Geometry check sheet. Reference: the model listing, model coordinates, mm. A direction names the side the tool comes from. Round coordinates to 2 decimals unless told otherwise and drop trailing zeros. Write each loop counter-clockwise with the first axis right and the second up, starting at its lowest first coordinate (ties: lowest second). Pieces come first, ordered by that corner, then holes.
Item 1: Depth check by flat-ended pin: P1, Ø3, axis at y = 14, z = -18.5, coming from the -X side; P2, Ø4.5, axis at y = 15, z = 20, coming from the +X side; P3, Ø8, axis at x = -10, y = 8, coming from the -Z side. Enter the tip coordinate at first touch or a pass-through.
Item 2: Access from +Z, -Z, +X, -X, +Y, -Y to the whole of each face (thin tool, end or side, straight path). Record for faces 4 (the face through (0, 13, 20)), 5 (the face through (1.5, 15, 20)), 6 (the face through (-1.5, 15, -20)), 7 (the face through (-3.3, 15, -3.3)).
Item 3: Cross-section at D-D (x = -13.5). Enter the section's corners in (y, z), then the cut area to 3 significant figures.
Item 4: Cross-section at C-C (y = 15.75). Enter the section's corners in (x, z), then the cut area to 3 significant figures.
Item 5: Cross-section at B-B (z = -2). Enter the section's corners in (x, y).
Item 6: Cross-section at A-A (x = 0). Enter the section's corners in (y, z).
Item 7: Draft check along X on faces 1 (the face through (-16, 8, 0)), 2 (the face through (0, 8, 16)), 3 (the face through (14, 7, 0)). Enter one of: pulls with the +X half, pulls with the -X half, needs draft (parallel to the pull), parting line crosses it, or undercut.
Item 8: Scan lines: probe 1 along Z at (x, y) = (8, 14.75); probe 2 along X at (y, z) = (16.3, 0). Record each from-to range of solid material in increasing order.
from build123d import *

# Parameters (mm, degrees)
SKETCH1_W           = 32
SKETCH1_H           = 32
SKETCH1_W_2         = 28
SKETCH1_H_2         = 28
BOSS_EXTRUDE1_DEPTH = 15
SKETCH2_W           = 32
SKETCH2_H           = 32
BOSS_EXTRUDE2_DEPTH = 2
CUT_EXTRUDE1_REACH  = 19
SKETCH3_R           = 4.25
SKETCH5_W           = 3
SKETCH5_H           = 4
BOSS_EXTRUDE3_DEPTH = 7.5


with BuildPart() as part:
    # Sketch1 → Boss-Extrude1 (new body)
    with BuildSketch(Plane(origin=(0, 0, 0), x_dir=(1, 0, 0), z_dir=(0, 1, 0))):
        Rectangle(SKETCH1_W, SKETCH1_H)
        Rectangle(SKETCH1_W_2, SKETCH1_H_2, mode=Mode.SUBTRACT)
    extrude(amount=BOSS_EXTRUDE1_DEPTH)

    # Sketch2 → Boss-Extrude2 (add)
    with BuildSketch(Plane(origin=(0, 15, 0), x_dir=(1, 0, 0), z_dir=(0, 1, 0))):
        Rectangle(SKETCH2_W, SKETCH2_H)
    extrude(amount=BOSS_EXTRUDE2_DEPTH)

    # Sketch3 → Cut-Extrude1 (cut, up to next)
    with BuildSketch(Plane(origin=(0, 17, 0), x_dir=(1, 0, 0), z_dir=(0, 1, 0)), mode=Mode.PRIVATE) as cut_extrude1_sk1:
        Circle(SKETCH3_R)
    cut_extrude1_tool1 = extrude(cut_extrude1_sk1.sketch, amount=-CUT_EXTRUDE1_REACH, mode=Mode.PRIVATE) & part.part
    add(cut_extrude1_tool1.solids().sort_by_distance((0, 17, 0))[0], mode=Mode.SUBTRACT)

    # Sketch5 → Boss-Extrude3 (add)
    with BuildSketch(Plane(origin=(0, 0, -16), x_dir=(-1, 0, 0), z_dir=(0, 0, -1))):
        with Locations((0, 15)):
            Rectangle(SKETCH5_W, SKETCH5_H)
    boss_extrude3 = extrude(amount=BOSS_EXTRUDE3_DEPTH)

    # Mirror1: Boss-Extrude3 across plane
    add(boss_extrude3.mirror(Plane.XY))


solid = part.part
Resolved:
1. P1: stops at x = -1.5
1. P2: stops at x = 1.5
1. P3: stops at z = -16
2. face 4: +Z, +X, -X, -Y
2. face 5: +Z, +X, +Y, -Y
2. face 6: -Z, -X, +Y, -Y
2. face 7: -Y
3. outline: (0, -16) - (17, -16) - (17, 16) - (0, 16) - (0, 14) - (15, 14) - (15, -14) - (0, -14) - close
3. area: 124 mm2
4. outline: (-16, -16) - (-1.5, -16) - (-1.5, -23.5) - (1.5, -23.5) - (1.5, -16) - (16, -16) - (16, 16) - (1.5, 16) - (1.5, 23.5) - (-1.5, 23.5) - (-1.5, 16) - (-16, 16) - close; hole circle Ø8.5 at (0, 0)
4. area: 1,010 mm2
5. outline: (-16, 0) - (-14, 0) - (-14, 15) - (-3.75, 15) - (-3.75, 17) - (-16, 17) - close; (3.75, 15) - (14, 15) - (14, 0) - (16, 0) - (16, 17) - (3.75, 17) - close
6. outline: (0, -16) - (13, -16) - (13, -23.5) - (17, -23.5) - (17, -4.25) - (15, -4.25) - (15, -14) - (0, -14) - close; (0, 14) - (15, 14) - (15, 4.25) - (17, 4.25) - (17, 23.5) - (13, 23.5) - (13, 16) - (0, 16) - close
7. face 1: pulls with the -X half
7. face 2: needs draft
7. face 3: undercut
8. probe 1: z = -16 to -14, 14 to 16
8. probe 2: x = -16 to -4.25, 4.25 to 16
